Here's how the part is built. I have some questions about the finished solid (model axes, mm). Face numbers are marked on the shaded views. A direction names the side the tool comes from. Give positions to 0.01 mm unless a question says otherwise; leave off trailing zeros. Order: outer loops, then holes, each group sorted by start corner. A loop starts at its lowest first (then second) coordinate and runs counter-clockwise, first axis right, second up.
from build123d import *

# Parameters (mm, degrees)
SKETCH1_W           = 50
SKETCH1_H           = 50
BOSS_EXTRUDE1_DEPTH = 89.61
SKETCH2_R           = 15
CUT_EXTRUDE1_DEPTH  = 97.332508013
SKETCH3_W           = 49.61
SKETCH3_H           = 30
CUT_EXTRUDE2_DEPTH  = 106.61700668
FILLET3_R           = 5
FILLET4_R           = 10
SKETCH4_R           = 5
CUT_EXTRUDE3_DEPTH  = 106.61700668


with BuildPart() as part:
    # Sketch1 → Boss-Extrude1 (new body)
    with BuildSketch(Plane.XY):
        Rectangle(SKETCH1_W, SKETCH1_H)
    extrude(amount=BOSS_EXTRUDE1_DEPTH)

    # Sketch2 → Cut-Extrude1 (cut, through all)
    with BuildSketch(Plane(origin=(0, 0, 0), x_dir=(-1, 0, 0), z_dir=(0, 0, -1))):
        Circle(SKETCH2_R)
    extrude(amount=-CUT_EXTRUDE1_DEPTH, mode=Mode.SUBTRACT)

    # Sketch3 → Cut-Extrude2 (cut, through all)
    with BuildSketch(Plane.ZY.offset(25)):
        with Locations((64.805, 0)):
            Rectangle(SKETCH3_W, SKETCH3_H)
    extrude(amount=-CUT_EXTRUDE2_DEPTH, mode=Mode.SUBTRACT)

    # Fillet3
    fillet3_edges = [part.edges().sort_by_distance(p)[0] for p in [
        (0, -25, 0),
        (-25, 0, 0),
        (0, 25, 0),
        (25, 0, 0),
    ]]
    fillet(fillet3_edges, radius=FILLET3_R)

    # Fillet4
    # the kernel refuses this fillet: 10 mm, written as the material it takes off along each edge
    with BuildSketch(Plane(origin=(-15, -15, 0), x_dir=(0, -1, 0), z_dir=(1, 0, 0))) as fillet4_piece_1:
        with BuildLine():
            CenterArc((5, -5), 5, 0, 90)
            Line((10, -5), (10, 0))
            Line((10, 0), (5, 0))
        make_face()
    revolve(axis=Axis((-15, -15, 0), (0, 0, -1)), revolution_arc=90, mode=Mode.SUBTRACT)
    with BuildSketch(Plane(origin=(15, -15, 0), x_dir=(1, 0, 0), z_dir=(0, 1, 0))) as fillet4_piece_2:
        with BuildLine():
            CenterArc((5, -5), 5, 0, 90)
            Line((10, -5), (10, 0))
            Line((10, 0), (5, 0))
        make_face()
    revolve(axis=Axis((15, -15, 0), (0, 0, -1)), revolution_arc=90, mode=Mode.SUBTRACT)
    with BuildSketch(Plane(origin=(15, 15, 0), x_dir=(0, 1, 0), z_dir=(-1, 0, 0))) as fillet4_piece_3:
        with BuildLine():
            CenterArc((5, -5), 5, 0, 90)
            Line((10, -5), (10, 0))
            Line((10, 0), (5, 0))
        make_face()
    revolve(axis=Axis((15, 15, 0), (0, 0, -1)), revolution_arc=90, mode=Mode.SUBTRACT)
    with BuildSketch(Plane(origin=(-15, 15, 0), x_dir=(-1, 0, 0), z_dir=(0, -1, 0))) as fillet4_piece_4:
        with BuildLine():
            CenterArc((5, -5), 5, 0, 90)
            Line((10, -5), (10, 0))
            Line((10, 0), (5, 0))
        make_face()
    revolve(axis=Axis((-15, 15, 0), (0, 0, -1)), revolution_arc=90, mode=Mode.SUBTRACT)
    with BuildSketch(Plane(origin=(-25, 25, 0), x_dir=(1, 0, 0), z_dir=(0, 0, 1)), Plane(origin=(-25, -25, 0), x_dir=(0, 1, 0), z_dir=(0, 0, 1))) as fillet4_piece_5:
        with BuildLine():
            CenterArc((FILLET4_R, -FILLET4_R), FILLET4_R, 90, 90)
            Line((0, -FILLET4_R), (0, 0))
            Line((0, 0), (FILLET4_R, 0))
        make_face()
    extrude(amount=114.61, mode=Mode.SUBTRACT)
    with BuildSketch(Plane(origin=(25, 25, 0), x_dir=(-1, 0, 0), z_dir=(0, 0, 1)), Plane(origin=(25, -25, 0), x_dir=(0, 1, 0), z_dir=(0, 0, 1))) as fillet4_piece_6:
        with BuildLine():
            CenterArc((FILLET4_R, FILLET4_R), FILLET4_R, 180, 90)
            Line((0, FILLET4_R), (0, 0))
            Line((0, 0), (FILLET4_R, 0))
        make_face()
    extrude(amount=114.61, mode=Mode.SUBTRACT)

    # Sketch4 → Cut-Extrude3 (cut, through all)
    with BuildSketch(Plane(origin=(0, 25, 0), x_dir=(1, 0, 0), z_dir=(0, 1, 0))):
        with Locations(Location((0, -75, 0), (0, 0, 270))):
            Circle(SKETCH4_R)
        with BuildLine():
            Line((-2.228917094, -89.61), (2.228917094, -89.61))
            ThreePointArc((2.228917094, -89.61), (4.246928068, -88.829826954), (5.21534053, -86.895087804))
            ThreePointArc((5.21534053, -86.895087804), (11.515192631, -61.931906551), (25, -40))
            add(Edge.make_bspline(
                [(-25, -40), (-88.150639052, -71.432998628), (-33.241224171, -142.040624048), (62.119232947, -121.01307169), (53.993290676, -50.260593277), (25, -40)],
                knots=[0, 0, 0, 0, 0.488610216, 0.657386139, 1, 1, 1, 1], degree=3))
            ThreePointArc((-25, -40), (-11.515192631, -61.931906551), (-5.21534053, -86.895087804))
            ThreePointArc((-5.21534053, -86.895087804), (-4.246928068, -88.829826954), (-2.228917094, -89.61))
        make_face()
    extrude(amount=-CUT_EXTRUDE3_DEPTH, mode=Mode.SUBTRACT)


solid = part.part
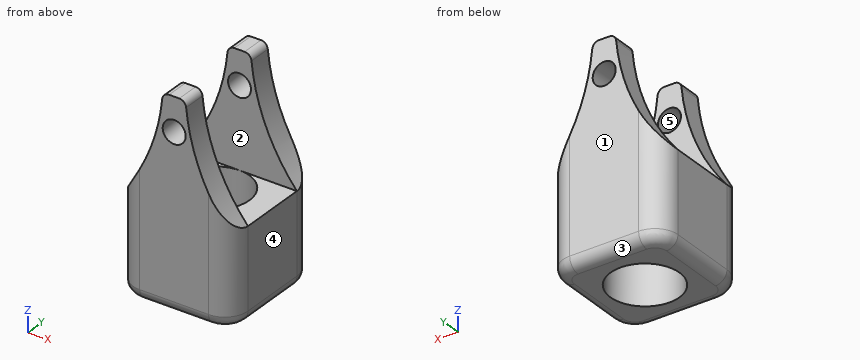
Q1. If we section it at B-B on x = -11: List the corners of the cut face in (y, z) for me.
Filled sheet:
outline: (-25, 5) arc R5 ccw to (-20, 0) - (-10.2, 0) - (-10.2, 40) - (-15, 40) - (-15, 63.18) - (-25, 63.18) - close; (10.2, 0) - (20, 0) arc R5 ccw to (25, 5) - (25, 63.18) - (15, 63.18) - (15, 40) - (10.2, 40) - close
Q2. For the marked faces 1 and 2, which set-ups out of +Z, -Z, +X, -X, +Y, -Y let a thin tool reach every point of the face, with its end or its side?
Filled sheet:
face 1: +Z, -Z, +X, -X, +Y
face 2: +Z, +X, -X
Q3. If we section it at D-D on y = -7.5: List the corners of the cut face in (x, z) for me, plus the area to 3 significant figures.
Filled sheet:
outline: (-25, 5) arc R5 ccw to (-20, 0) - (-12.99, 0) - (-12.99, 40) - (-25, 40) - close; (12.99, 0) - (20, 0) arc R5 ccw to (25, 5) - (25, 40) - (12.99, 40) - close
area: 950 mm2
Q4. Thinking about a two-plate mould opening in X: for the marked faces 3, 4 and 5, which applies, released by +X, released by -X, zero draft, split by the parting line, or undercut?
Filled sheet:
face 3: zero draft
face 4: released by +X
face 5: undercut
Q5. If we section it at C-C on z = 83.5: List the corners of the cut face in (x, y) for me.
Filled sheet:
outline: (-5.61, -25) - (5.61, -25) - (5.61, -15) - (-5.61, -15) - close; (-5.61, 15) - (5.61, 15) - (5.61, 25) - (-5.61, 25) - close
Q6. I'm going to push flat-ended pins straight in: P1, Ø10, axis at x = 2.5, y = 9.5, coming from the -Z side; P2, Ø12.5, axis at x = 15.5, y = -2, coming from the +Z side; P3, Ø8, axis at y = -14, z = 48, coming from the +X side. Where does each tip first touch, or does it pass through?
Filled sheet:
P1: passes through
P2: stops at z = 40
P3: stops at x = 21.72
Q7. I need wall thicknesses on L1, parallel to Y at x = -11.5, z = 52; L2, parallel to Y at x = 11, z = 19; L3, parallel to Z at x = 11.5, y = 14. Which ranges of each line are inside material? Lowest first, please.
Filled sheet:
L1: y = -25 to -15, 15 to 25
L2: y = -25 to -10.2, 10.2 to 25
L3: z = 0 to 40
Q8. If we section it at A-A on y = 0: List the corners of the cut face in (x, z) for me, plus the area to 3 significant figures.
Filled sheet:
outline: (-25, 5) arc R5 ccw to (-20, 0) - (-15, 0) - (-15, 40) - (-25, 40) - close; (15, 0) - (20, 0) arc R5 ccw to (25, 5) - (25, 40) - (15, 40) - close
area: 789 mm2
